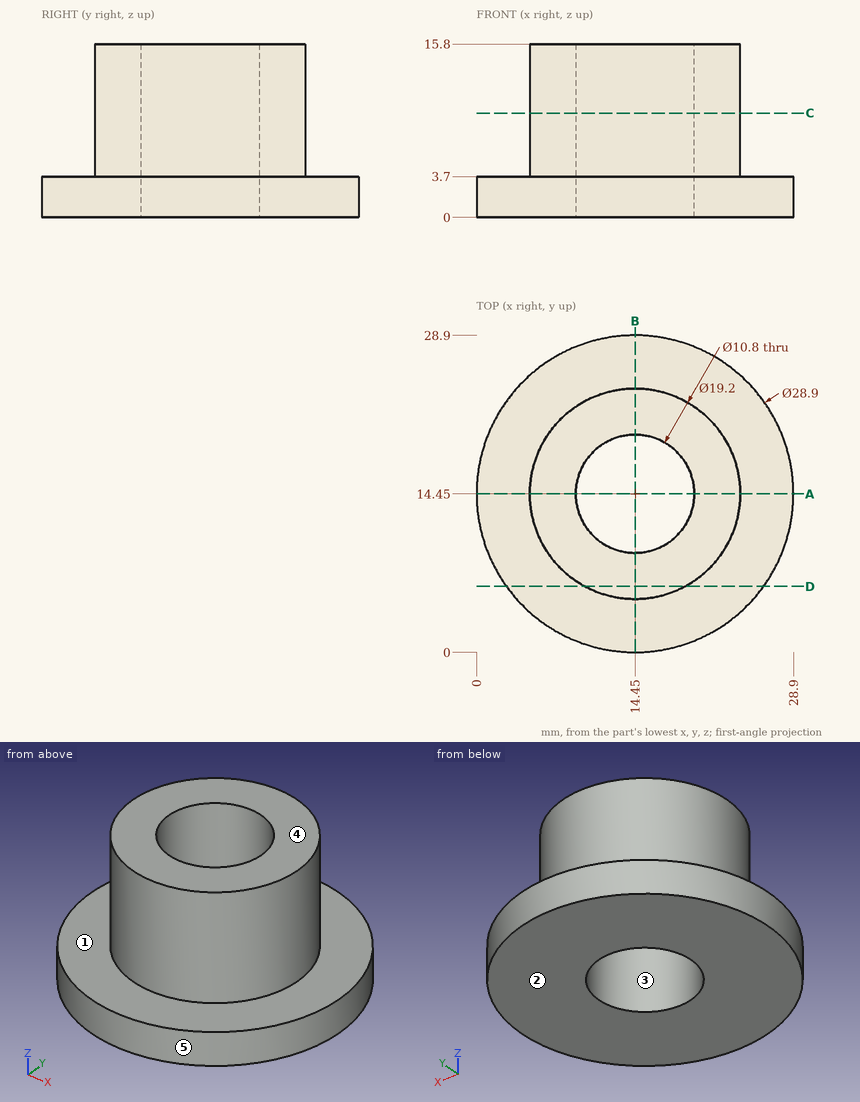
Drawing for the job (mm, zero at the part's lowest x, y, z). A direction names the side the tool comes from. Round coordinates to 2 decimals unless told otherwise and drop trailing zeros. Write each loop counter-clockwise with the first axis right and the second up, starting at its lowest first coordinate (ties: lowest second). Pieces come first, ordered by that corner, then holes. Notation, with made-up numbers: (-1, 73) - (31, 73) arc R9 cw to (31, 82) - close; hole circle Ø5 at (-40, 15.5). An arc over 180 degrees is marked (long way). Write item = value, one per line. Start each with the question number.
Q1. Band-saw the part on C-C (z = 9.5). Give the cut face in (x, y), then the cut area to 3 significant figures.
Q2. Probe L1, parallel to X at y = 14.45, z = 7.25; L2, parallel to Z at x = 21.5, y = 2.75. List the from-to ranges inside material, lowest first. Write a range as from..to.
Q3. Mould opens along Y. For the marked faces 3, 4 and 5 say: pulls with the +Y half, pulls with the -Y half, needs draft (parallel to the pull), parting line crosses it, or undercut.
Q4. Band-saw the part on A-A (y = 14.45). Give the cut face in (x, z), then the cut area to 3 significant figures.
Q5. Which spindle directions (+Z, -Z, +X, -X, +Y, -Y) get a long thin tool onto all of the face, cutting with end or side? Do the marked faces 1 and 2. Say none if no direction does.
Q6. Drop flat-ended pins along their axis: pin 1 (1.5 mm diameter, centred on y = 21, z = 7.5, fed in from -X); pin 2 (5 mm diameter, centred on x = 25, y = 8, fed in from +Z); pin 3 (1 mm diameter, centred on y = 13, z = 7.5, fed in from +X); pin 4 (3 mm diameter, centred on x = 17.5, y = 16, fed in from -Z). Give the stop position or say it passes through.
Q7. Band-saw the part on D-D (y = 6). Give the cut face in (x, z).
Answers below:
q1.outline = circle Ø19.2 at (14.45, 14.45); hole circle Ø10.8 at (14.45, 14.45)
q1.area = 198 mm2
q2.L1 = 4.85..9.05, 19.85..24.05
q2.L2 = 0..3.7
q3.face_3 = undercut
q3.face_4 = needs draft
q3.face_5 = parting line crosses it
q4.outline = (0, 0) - (9.05, 0) - (9.05, 15.8) - (4.85, 15.8) - (4.85, 3.7) - (0, 3.7) - close; (19.85, 0) - (28.9, 0) - (28.9, 3.7) - (24.05, 3.7) - (24.05, 15.8) - (19.85, 15.8) - close
q4.area = 169 mm2
q5.face_1 = +Z
q5.face_2 = -Z, +X, -X, +Y, -Y
q6.pin_1 = 6.8
q6.pin_2 = 3.7
q6.pin_3 = 24
q6.pin_4 = through
q7.outline = (2.73, 0) - (26.17, 0) - (26.17, 3.7) - (19.01, 3.7) - (19.01, 15.8) - (9.89, 15.8) - (9.89, 3.7) - (2.73, 3.7) - close
